from build123d import *

# Parameters (mm, degrees)
CROQUIS3_R              = 1.2
CROQUIS3_R_2            = 0.95
SALIENTE_EXTRUIR4_DEPTH = 1.6
REDONDEO4_R             = 0.5
REDONDEO5_R             = 0.5


with BuildPart() as part:
    # Croquis3 → Saliente-Extruir4 (new body)
    with BuildSketch(Plane.XY):
        Polygon((4.131159953, -85.774171861), (10.73555349, 15.325828139), (-1.049372117, 17.587581538), (-7.653765654, -83.512418462), align=None)
        with Locations((4.843090686, 12.756704839)):
            Circle(CROQUIS3_R, mode=Mode.SUBTRACT)
        with Locations((4.450627883, 6.677578183)):
            Circle(CROQUIS3_R, mode=Mode.SUBTRACT)
        with Locations((-1.611374093, -82.348187023)):
            Circle(CROQUIS3_R_2, mode=Mode.SUBTRACT)
    extrude(amount=SALIENTE_EXTRUIR4_DEPTH)

    # Redondeo4
    redondeo4_edges = [part.edges().sort_by_distance(p)[0] for p in [
        (10.73555349, 15.325828139, 0.8),
    ]]
    fillet(redondeo4_edges, radius=REDONDEO4_R)

    # Redondeo5
    redondeo5_edges = [part.edges().sort_by_distance(p)[0] for p in [
        (4.131159953, -85.774171861, 0.8),
        (-7.653765654, -83.512418462, 0.8),
        (-1.049372117, 17.587581538, 0.8),
    ]]
    fillet(redondeo5_edges, radius=REDONDEO5_R)


solid = part.part
The listing builds one solid part. Answer for the finished solid, in the listing's coordinates (mm). Give positions to 0.01 mm unless a question says otherwise; leave off trailing zeros. Order: outer loops, then holes, each group sorted by start corner. A loop starts at its lowest first (then second) coordinate and runs counter-clockwise, first axis right, second up. Notation, with made-up numbers: (81.5, 85.5) - (97.5, 85.5) arc R27 cw to (97.5, 119.5) - close; hole circle Ø3 at (83, -28.75). An arc over 180 degrees is marked (long way). Answer as CSV lines item,"result".
Q1. A cutting plane is placed at C-C, the plane y = -42. Determine the outline of the cut face in (x, z).
Answer key:
outline,"(-4.94, 0) - (6.99, 0) - (6.99, 1.6) - (-4.94, 1.6) - close"
Q2. A cutting plane is placed at A-A, the plane z = 0.65. Determine the outline of the cut face in (x, y) (3 decimals), and give its area (3 significant figures).
Answer key:
outline,"(-7.625, -83.072) arc R0.5 ccw to (-7.22, -83.596) - (3.575, -85.667) arc R0.5 ccw to (4.168, -85.209) - (10.707, 14.885) arc R0.5 ccw to (10.302, 15.409) - (-0.493, 17.481) arc R0.5 ccw to (-1.086, 17.022) - close; hole circle Ø1.9 at (-1.611, -82.348); hole circle Ø2.4 at (4.451, 6.678); hole circle Ø2.4 at (4.843, 12.757)"
area,"1,190 mm^2"
Q3. Straight lines are drawn through the part: L1, parallel to Y at x = 4, z = 1.1; L2, parallel to Y at x = -1, z = 0.25; L3, parallel to Y at x = 0, z = 1.1. For each, find the intervals that lie inside material, in ascending order.
Answer key:
L1,"y = -85.55 to 5.57, 7.79 to 11.9, 13.61 to 16.62"
L2,"y = -84.79 to -83.08, -81.62 to 17.27"
L3,"y = -84.98 to 17.39"
Q4. Determine the mould class of faces 1 (the face through (-1.898, -84.617, 0.789)), 2 (the face through (5, 5.61, 0.79)), 3 (the face through (-4.31, -32.32, 0.79)) for opening direction Y: pulls with the +Y half, pulls with the -Y half, needs draft (parallel to the pull), parting line crosses it, or undercut.
Answer key:
face 1,"pulls with the -Y half"
face 2,"undercut"
face 3,"pulls with the +Y half"
Q5. A cutting plane is placed at B-B, the plane x = -4.25. Determine the outline of the cut face in (y, z), and give its area (3 significant figures).
Answer key:
outline,"(-84.17, 0) - (-31.41, 0) - (-31.41, 1.6) - (-84.17, 1.6) - close"
area,"84.4 mm^2"
